from build123d import *

# Parameters (mm, degrees)
PAD_DEPTH    = 3
SKETCH001_R  = 1.5
PAD001_DEPTH = 6
SKETCH002_R  = 2.1
POCKET_DEPTH = 2
SKETCH003_R  = 3
PAD002_DEPTH = 3
FILLET_R     = 2.5


with BuildPart() as part:
    # Sketch → Pad (new body)
    with BuildSketch(Plane.XY):
        Polygon((-11.75, -33), (11.75, -33), (11.75, -11.5), (7, -11.5), (7, 33), (4, 33), (4, 43), (-4, 43), (-4, 33), (-7, 33), (-7, -11.5), (-11.75, -11.5), align=None)
    extrude(amount=PAD_DEPTH)

    # Sketch001 → Pad001 (join, symmetric)
    with BuildSketch(Plane.YZ):
        with Locations((40, 1.5)):
            Circle(SKETCH001_R)
    extrude(amount=PAD001_DEPTH, both=True)

    # Sketch002 (on Face5 of Pad001) → Pocket (cut)
    with BuildSketch(Plane.XY.offset(3)):
        with Locations((0, -23)):
            Circle(SKETCH002_R)
    extrude(amount=-POCKET_DEPTH, mode=Mode.SUBTRACT)

    # Sketch003 (on Face5 of Pocket) → Pad002 (join)
    with BuildSketch(Plane.XY.offset(3)):
        with Locations((0, 23)):
            Circle(SKETCH003_R)
    extrude(amount=PAD002_DEPTH)

    # Fillet
    fillet_edges = [part.edges().sort_by_distance(p)[0] for p in [
        (-3, 23, 6),
    ]]
    fillet(fillet_edges, radius=FILLET_R)


solid = part.part
The model under review builds one solid part; all positions refer to its coordinate system, in mm. A direction names the side the tool comes from. Round coordinates to 2 decimals unless told otherwise and drop trailing zeros. Loops run counter-clockwise (first coordinate to the right, second up) from the corner with the lowest first, then second, coordinate; pieces in that order, holes last. Notation, with made-up numbers: (3, -35.5) -> (35, -35.5) arc R32 ccw to (35, -3.5) -> close; hole circle Ø8 at (-9.5, -10.75). An arc over 180 degrees is marked (long way). Write item = value, one per line. Start each with the question number.
Item 1: Take a section at B-B on x = -9.5. Give the boundary of the cut face in (y, z).
Item 2: Take a section at C-C on y = 3. Give the boundary of the cut face in (x, z).
Item 3: To check wall thickness, follow L1, parallel to Y at x = 0, z = 1.75; L2, parallel to Y at x = 10.5, z = 1.9; L3, parallel to Z at x = -5, y = 21. State the ranges of each line that lie inside material, in increasing order.
Item 4: Take a section at A-A on y = -23. Give the boundary of the cut face in (x, z), plus the area to 3 significant figures.
Item 5: Mouldability with a two-part tool opening along Y and no side actions: class faces 1 (the flat face through (7, 10, 1)), 2 (the cylindrical face through (5.01, 38.5, 1.57)), 3 (the cylindrical face through (-0.65, 20.07, 3.25)) as released by +Y, released by -Y, zero draft, split by the parting line, or undercut.
Item 6: Insertion check: pin 1 (1.5 mm diameter, centred on y = 41, z = 2, fed in from +X); pin 2 (3.5 mm diameter, centred on y = 8.5, z = 1.5, fed in from +X); pin 3 (1.5 mm diameter, centred on x = 6, z = 2, fed in from +Y). Each pin has a flat end and moves straight along its axis. Give the tip position at first contact, or say it passes through.
Item 7: For faces 4 (the flat face through (-5, 33, 1)), 5 (the flat face through (0, -23, 1)), 6 (the flat face through (4, 42, 1)), list the 3-axis set-ups (+Z, -Z, +X, -X, +Y, -Y) from which the entire face can be reached by the end or side of a thin tool; tool diameter is ignored.
Result:
q1.outline = (-33, 0) -> (-11.5, 0) -> (-11.5, 3) -> (-33, 3) -> close
q2.outline = (-7, 0) -> (7, 0) -> (7, 3) -> (-7, 3) -> close
q3.L1 = -33 to -25.1, -20.9 to 43
q3.L2 = -33 to -11.5
q3.L3 = 0 to 3
q4.outline = (-11.75, 0) -> (11.75, 0) -> (11.75, 3) -> (2.1, 3) -> (2.1, 1) -> (-2.1, 1) -> (-2.1, 3) -> (-11.75, 3) -> close
q4.area = 62.1 mm²
q5.face_1 = zero draft
q5.face_2 = undercut
q5.face_3 = split by the parting line
q6.pin_1 = 6
q6.pin_2 = 7
q6.pin_3 = 41.5
q7.face_4 = +Z, -Z, -X
q7.face_5 = +Z
q7.face_6 = +X, +Y
